Could you check a few things on this drawing? It's one solid part, dimensions in mm from its lowest x, y, z. Round coordinates to 2 decimals unless told otherwise and drop trailing zeros. Write each loop counter-clockwise with the first axis right and the second up, starting at its lowest first coordinate (ties: lowest second). Pieces come first, ordered by that corner, then holes. Notation, with made-up numbers: (25, 24.5) -> (61, 24.5) arc R16 ccw to (61, 30.5) -> close; hole circle Ø10 at (-12.75, 58). An arc over 180 degrees is marked (long way). Answer in a Markdown table with one row per item. Add a question column.
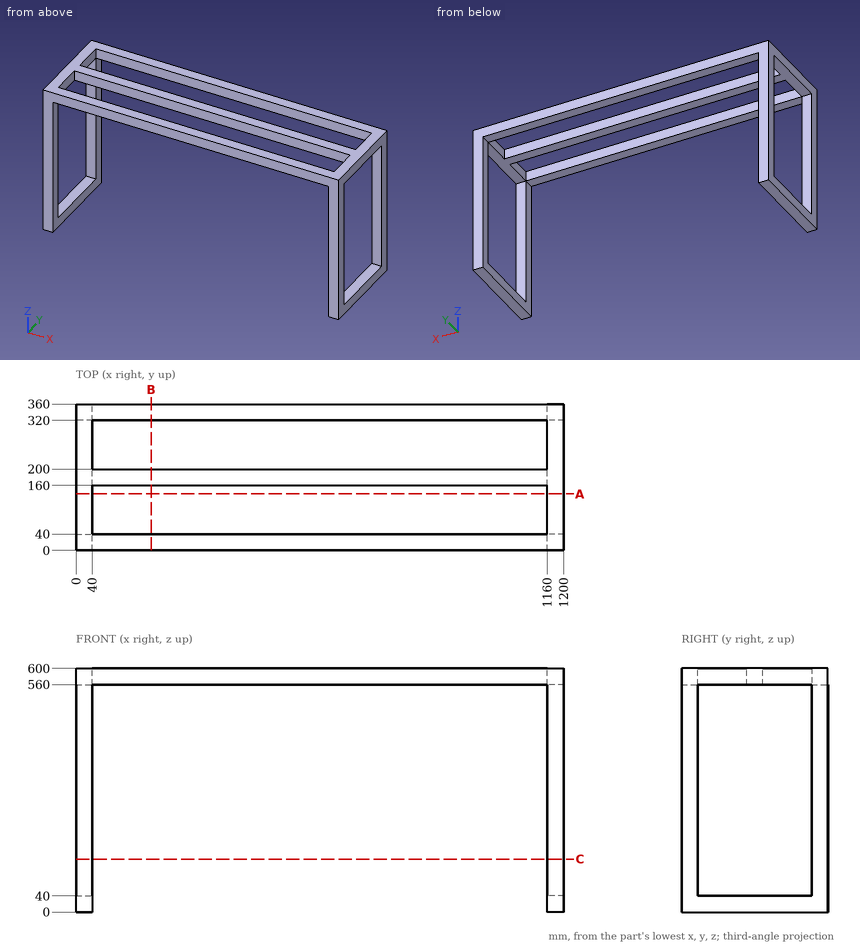
Item 1: For P1, Ø20, axis at x = 733.5, y = 346.5, coming from the -Z side, with a flat end and sliding along its axis, tell me the tip position at first contact or that it passes through.
Item 2: If we section it at C-C on z = 130.5: Please give me the cut outline in (x, y), then the cut area to 3 significant figures.
Item 3: If we section it at A-A on y = 139: Please give me the cut outline in (x, z).
Item 4: I need wall thicknesses on line 1 along X through (y, z) = (337, 466); line 2 along Z through (x, y) = (84.5, 338.5). Which ranges of each line are inside material? Lowest first, please. Write a range as from..to.
Item 5: If we section it at B-B on x = 185: Please give me the cut outline in (y, z).
Results list:
| question | item | result |
|---|---|---|
| 1 | P1 | z = 560 |
| 2 | outline | (0, 0) -> (40, 0) -> (40, 40) -> (0, 40) -> close; (0, 320) -> (40, 320) -> (40, 360) -> (0, 360) -> close; (1160, 0) -> (1200, 0) -> (1200, 40) -> (1160, 40) -> close; (1160, 320) -> (1200, 320) -> (1200, 360) -> (1160, 360) -> close |
| 2 | area | 6,400 mm² |
| 3 | outline | (0, 0) -> (40, 0) -> (40, 40) -> (0, 40) -> close; (0, 560) -> (40, 560) -> (40, 600) -> (0, 600) -> close; (1160, 0) -> (1200, 0) -> (1200, 40) -> (1160, 40) -> close; (1160, 560) -> (1200, 560) -> (1200, 600) -> (1160, 600) -> close |
| 4 | line 1 | 0..40, 1160..1200 |
| 4 | line 2 | 560..600 |
| 5 | outline | (0, 560) -> (40, 560) -> (40, 600) -> (0, 600) -> close; (160, 560) -> (200, 560) -> (200, 600) -> (160, 600) -> close; (320, 560) -> (360, 560) -> (360, 600) -> (320, 600) -> close |
